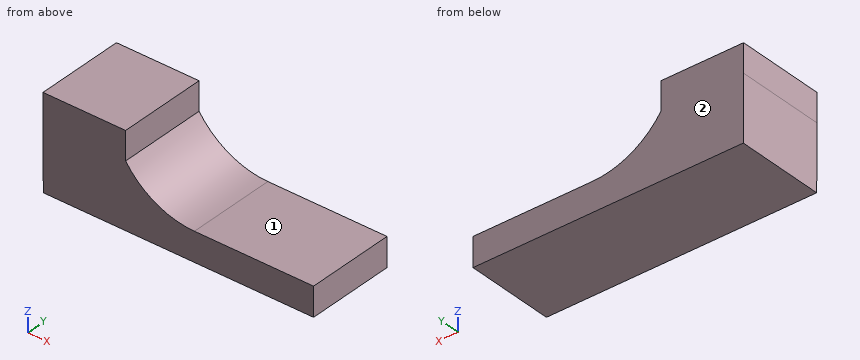
```python
from build123d import *

# Parameters (mm, degrees)
F0_W     = 119.03533
F0_H     = 28.961802
F0_W_2   = 82.531182
F0_H_2   = 28.334502
F1_DEPTH = 63.5
F2_DEPTH = 38.1


with BuildPart() as f1:
    # F0 (on Front) → F1 (new body, symmetric)
    with BuildSketch(Plane.XZ):
        Rectangle(F0_W, F0_H)
        with BuildLine():
            Line((-59.517665, -14.480901), (-59.517665, 14.480901))
            ThreePointArc((-59.517665, 14.480901), (-98.261712, 23.976224), (-128.224785, 50.310169))
            Line((-128.224785, 50.310169), (-210.755967, 50.310169))
            Line((-210.755967, 50.310169), (-210.454815, -14.480901))
            Line((-210.454815, -14.480901), (-59.517665, -14.480901))
        make_face()
        with Locations((-169.490376, 64.47742)):
            Rectangle(F0_W_2, F0_H_2)
    extrude(amount=F1_DEPTH, both=True)

    # F1_face (on face) → F2 (cut)
    with BuildSketch(Plane(origin=(-113.343632, 63.5, 19.109713), x_dir=(1, 0, 0), z_dir=(0, 1, 0))):
        with BuildLine():
            Line((172.861297, 4.628812), (172.861297, 33.590614))
            Line((172.861297, 33.590614), (-97.111183, 33.590614))
            Line((-97.111183, 33.590614), (-97.412335, -31.200456))
            Line((-97.412335, -31.200456), (-97.412335, -59.534958))
            Line((-97.412335, -59.534958), (-14.881153, -59.534958))
            Line((-14.881153, -59.534958), (-14.881153, -31.200456))
            ThreePointArc((-14.881153, -31.200456), (15.08192, -4.866511), (53.825967, 4.628812))
            Line((53.825967, 4.628812), (172.861297, 4.628812))
        make_face()
        with BuildLine():
            Line((-97.111183, 33.590614), (172.861297, 33.590614))
            Line((172.861297, 33.590614), (172.861297, 4.628812))
            Line((172.861297, 4.628812), (53.825967, 4.628812))
            ThreePointArc((53.825967, 4.628812), (15.08192, -4.866511), (-14.881153, -31.200456))
            Line((-14.881153, -31.200456), (-14.881153, -59.534958))
            Line((-14.881153, -59.534958), (-97.412335, -59.534958))
            Line((-97.412335, -59.534958), (-97.412335, -31.200456))
            Line((-97.412335, -31.200456), (-97.111183, 33.590614))
        make_face()
    extrude(amount=-F2_DEPTH, mode=Mode.SUBTRACT)


solid = f1.part
```
Source: CAD feature listing. Evaluate the final solid. Frame: model axes, mm. Face numbers are marked on the shaded views. A direction names the side the tool comes from. Round coordinates to 2 decimals unless told otherwise and drop trailing zeros. Loops run counter-clockwise (first coordinate to the right, second up) from the corner with the lowest first, then second, coordinate; pieces in that order, holes last. Notation, with made-up numbers: M 13.5,43.25 L 61.5,43.25 A20 cw 61.5,70.25 Z; hole C 49.5,65 d5. An arc over 180 degrees is marked long. Use a Markdown table: item, result. Add a question column.
1. Cut plane A-A, the plane y = -46.5. Output: boundary loops of the cut face in (x, z).
2. Cut plane B-B, the plane x = 2. Output: boundary loops of the cut face in (y, z), and give its area (3 significant figures).
3. Cut plane C-C, the plane z = 56.5. Output: boundary loops of the cut face in (x, y), and give its area (3 significant figures).
4. Contact query for flat-ended pins moving along their axis: pin 1 (2 mm diameter, centred on x = -18, y = -27, fed in from +Z); pin 2 (6 mm diameter, centred on x = -82.5, y = -48.5, fed in from +Z); pin 3 (22.5 mm diameter, centred on y = 0.5, z = 63, fed in from +X). Output: stop coordinate, or through.
5. Set-up query: the marked faces 1 and 2. Return all of +Z, -Z, +X, -X, +Y, -Y with unobstructed straight access to the full face (end or side cutting, diameter ignored); none if empty.
6. Ray query, line 1 along Z through (x, y) = (1.5, -36); line 2 along X through (y, z) = (-50, 51.5); line 3 along X through (y, z) = (-19, 8.5). Return the intervals inside material, ascending. Write a range as [from, to].
Solution:
| question | item | result |
|---|---|---|
| 1 | outline | M -210.76,50.31 L -210.45,-14.48 L 59.52,-14.48 L 59.52,14.48 L -59.52,14.48 A83.79 cw -128.22,50.31 L -128.22,78.64 L -210.76,78.64 Z |
| 2 | outline | M -63.5,-14.48 L 25.4,-14.48 L 25.4,14.48 L -63.5,14.48 Z |
| 2 | area | 2,570 mm2 |
| 3 | outline | M -210.76,-63.5 L -128.22,-63.5 L -128.22,25.4 L -210.76,25.4 Z |
| 3 | area | 7,340 mm2 |
| 4 | pin 1 | stops at z = 14.48 |
| 4 | pin 2 | stops at z = 18.61 |
| 4 | pin 3 | stops at x = -128.22 |
| 5 | face 1 | +Z, +X, +Y, -Y |
| 5 | face 2 | +Z, -Z, +X, -X, +Y |
| 6 | line 1 | z = [-14.48, 14.48] |
| 6 | line 2 | x = [-210.76, -128.22] |
| 6 | line 3 | x = [-210.56, 59.52] |
